Input: part model. Units: mm. Frame: model coordinates. Face numbers are marked on the shaded views. A direction names the side the tool comes from. Round coordinates to 2 decimals unless told otherwise and drop trailing zeros. Loops run counter-clockwise (first coordinate to the right, second up) from the corner with the lowest first, then second, coordinate; pieces in that order, holes last. Notation, with made-up numbers: (82, -31) - (99, -31) arc R33 ccw to (99, 7) - close; hole circle Ø9 at (18.25, -15). An arc over 180 degrees is marked (long way). One line per question, with ' | ' between items. Start each with the question number.
Item 1: Draft query along X for the marked faces 1, 2 and 3. Return one class per face: pulls with the +X half, pulls with the -X half, needs draft (parallel to the pull), parting line crosses it, or undercut.
Item 2: Set-up query: the marked faces 4, 5 and 6. Return all of +Z, -Z, +X, -X, +Y, -Y with unobstructed straight access to the full face (end or side cutting, diameter ignored); none if empty.
Item 3: Material intervals for line 1 along Z through (x, y) = (18.47, -7.75); line 2 along Z through (x, y) = (-38.8, -3.5); line 3 along Z through (x, y) = (28, -3.25), sorted ascending.
Item 4: Section B-B, the plane z = -16.5. Return loops of the section in (x, y).
Item 5: Section C-C, the plane y = -15.5. Return loops of the section in (x, z), plus the area to 3 significant figures.
Item 6: First-contact query: pin 1 (3 mm diameter, centred on x = 36, z = 1, fed in from -Y); pin 2 (1.8 mm diameter, centred on x = -10.5, z = 26.5, fed in from -Y). Flat tips, straight axial feed; report the tip coordinate or a pass-through.
Item 7: Section D-D, the plane y = -5.75. Give the number of separate pieces and of enclosed holes in the cut face, plus the area to 3 significant figures.
Item 8: Section A-A, the plane x = -16. Return loops of the section in (y, z).
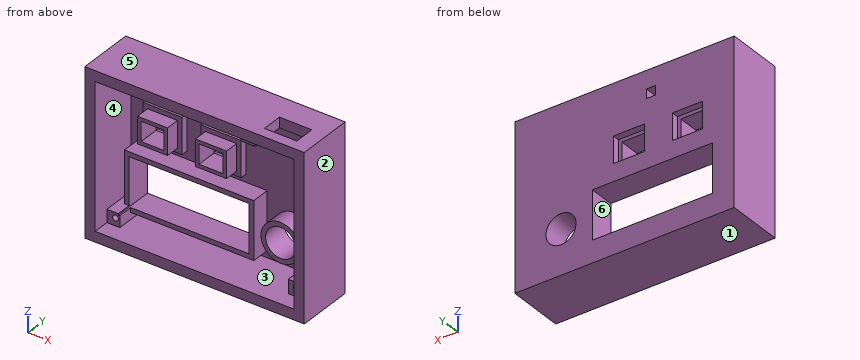
```python
from build123d import *

# Parameters (mm, degrees)
SKETCH1_W             = 13
SKETCH1_H             = 11.5
SKETCH1_W_2           = 13.406613497
SKETCH1_W_3           = 52
SKETCH1_H_2           = 21
SKETCH1_R             = 6.5
BOSS_EXTRUDE1_DEPTH   = 3
SKETCH2_W             = 95
SKETCH2_H             = 71.500049505
BOSS_EXTRUDE2_DEPTH   = 21.5
SKETCH3_R             = 1.25
SKETCH3_W             = 7.478374846
SKETCH3_H             = 5.979454016
SKETCH3_W_2           = 5.973627986
SKETCH3_H_2           = 6.528755861
BOSS_EXTRUDE3_DEPTH   = 14.5
CUT_EXTRUDE1_REACH    = 73.5
SKETCH4_W             = 14
SKETCH4_H             = 9
SKETCH5_R             = 8.5
SKETCH5_R_2           = 6.5
SKETCH5_W             = 56
SKETCH5_H             = 25
SKETCH5_W_2           = 52
SKETCH5_H_2           = 21
BOSS_EXTRUDE4_DEPTH   = 8
SKETCH7_W             = 6
SKETCH7_H             = 6
SKETCH7_W_2           = 4
SKETCH7_H_2           = 4
BOSS_EXTRUDE5_DEPTH   = 13
SKETCH8_W             = 10
SKETCH8_H             = 8.5
BOSS_EXTRUDE6_DEPTH   = 9
SKETCH8_W_2           = 13.406613497
SKETCH8_H_2           = 11.5
SKETCH8_W_3           = 10.406613497
BOSS_EXTRUDE6_2_DEPTH = 9
SKETCH9_W             = 17.406613497
SKETCH9_H             = 15.5
SKETCH9_W_2           = 13.406613497
SKETCH9_H_2           = 11.5
SKETCH9_W_3           = 17
SKETCH9_W_4           = 13
BOSS_EXTRUDE7_DEPTH   = 3
CUT_EXTRUDE2_DEPTH    = 5


with BuildPart() as part:
    # Sketch1 → Boss-Extrude1 (new body)
    with BuildSketch(Plane(origin=(0, 0, 0), x_dir=(1, 0, 0), z_dir=(0, 1, 0))):
        Polygon((48, 35.75), (46, 35.75), (45, 35.75), (-47, 35.75), (-47, 33.75), (-47, -33.75), (-47, -35.750049505), (45, -35.750049505), (46, -35.750049505), (48, -35.750049505), align=None)
        Polygon((-8, -29), (-11, -29), (-14, -29), (-14, -23), (-8, -23), align=None, mode=Mode.SUBTRACT)
        with Locations((-26.716961343, -8)):
            Rectangle(SKETCH1_W, SKETCH1_H, mode=Mode.SUBTRACT)
        with Locations((-1.396693251, -8)):
            Rectangle(SKETCH1_W_2, SKETCH1_H, mode=Mode.SUBTRACT)
        with Locations((-11.6, 15.75)):
            Rectangle(SKETCH1_W_3, SKETCH1_H_2, mode=Mode.SUBTRACT)
        with Locations((28, 16.5)):
            Circle(SKETCH1_R, mode=Mode.SUBTRACT)
    extrude(amount=BOSS_EXTRUDE1_DEPTH)

    # Sketch2 → Boss-Extrude2 (add)
    with BuildSketch(Plane.XZ):
        with Locations((0.5, 2.4752e-05)):
            Rectangle(SKETCH2_W, SKETCH2_H)
        Polygon((41.5, -31.25), (40.5, -31.25), (-42.5, -31.25), (-42.5, 31.25), (40.5, 31.25), (41.5, 31.25), (43.5, 31.25), (43.5, -31.25), align=None, mode=Mode.SUBTRACT)
    extrude(amount=BOSS_EXTRUDE2_DEPTH)

    # Sketch3 → Boss-Extrude3 (add)
    with BuildSketch(Plane.XZ):
        Polygon((-38.8, -25.675777927), (-42.5, -25.675777927), (-42.5, -31.25), (-36.902935229, -31.25), (-36.902935229, -27.93), (-36.902935229, -26.25), (-37.6, -26.25), (-37.6, -25.675777927), align=None)
        with Locations((-38.8, -27.93)):
            Circle(SKETCH3_R, mode=Mode.SUBTRACT)
        with Locations((39.760812577, -28.260272992)):
            Rectangle(SKETCH3_W, SKETCH3_H)
        with Locations((39.43, -27.68)):
            Circle(SKETCH3_R, mode=Mode.SUBTRACT)
        with Locations((18.554223867, 27.98562207)):
            Rectangle(SKETCH3_W_2, SKETCH3_H_2)
        with Locations((18.47, 27.69)):
            Circle(SKETCH3_R, mode=Mode.SUBTRACT)
    extrude(amount=BOSS_EXTRUDE3_DEPTH)

    # Sketch4 → Cut-Extrude1 (cut, up to next)
    with BuildSketch(Plane.XY.offset(35.750049505), mode=Mode.PRIVATE) as cut_extrude1_sk1:
        with Locations((34.5, -12.5)):
            Rectangle(SKETCH4_W, SKETCH4_H)
    cut_extrude1_tool1 = extrude(cut_extrude1_sk1.sketch, amount=-CUT_EXTRUDE1_REACH, mode=Mode.PRIVATE) & part.part
    add(cut_extrude1_tool1.solids().sort_by_distance((34.5, -12.5, 35.75005))[0], mode=Mode.SUBTRACT)

    # Sketch5 → Boss-Extrude4 (add)
    with BuildSketch(Plane.XZ):
        with Locations((28, -16.5)):
            Circle(SKETCH5_R)
        with Locations((28, -16.5)):
            Circle(SKETCH5_R_2, mode=Mode.SUBTRACT)
        with Locations((-11.6, -15.75)):
            Rectangle(SKETCH5_W, SKETCH5_H)
        with Locations((-11.6, -15.75)):
            Rectangle(SKETCH5_W_2, SKETCH5_H_2, mode=Mode.SUBTRACT)
    extrude(amount=BOSS_EXTRUDE4_DEPTH)

    # Sketch7 → Boss-Extrude5 (add)
    with BuildSketch(Plane(origin=(0, 3, 0), x_dir=(1, 0, 0), z_dir=(0, 1, 0))):
        with Locations((-11, -26)):
            Rectangle(SKETCH7_W, SKETCH7_H)
        with Locations((-11, -26)):
            Rectangle(SKETCH7_W_2, SKETCH7_H_2, mode=Mode.SUBTRACT)
    extrude(amount=-BOSS_EXTRUDE5_DEPTH)



with BuildPart() as body_2:
    # Sketch8 → Boss-Extrude6 (new body)
    with BuildSketch(Plane.XZ):
        Polygon((-33.216961343, 12.25), (-33.216961343, 2.25), (-20.216961343, 2.25), (-20.216961343, 12.25), (-20.216961343, 13.75), (-33.216961343, 13.75), align=None)
        with Locations((-26.716961343, 8)):
            Rectangle(SKETCH8_W, SKETCH8_H, mode=Mode.SUBTRACT)
    extrude(amount=BOSS_EXTRUDE6_DEPTH)


with BuildPart() as body_3:
    # Sketch8 → Boss-Extrude6 2 (new body)
    with BuildSketch(Plane.XZ):
        with Locations((-1.396693251, 8)):
            Rectangle(SKETCH8_W_2, SKETCH8_H_2)
        with Locations((-1.396693252, 8)):
            Rectangle(SKETCH8_W_3, SKETCH8_H, mode=Mode.SUBTRACT)
    extrude(amount=BOSS_EXTRUDE6_2_DEPTH)


with BuildPart() as part_1:
    add(part.part)

    add(body_2.part)  # Boss-Extrude7 merges body 2

    add(body_3.part)  # Boss-Extrude7 merges body 3
    # Sketch9 → Boss-Extrude7 (add)
    with BuildSketch(Plane.XZ):
        with Locations((-1.396693252, 8)):
            Rectangle(SKETCH9_W, SKETCH9_H)
        with Locations((-1.396693251, 8)):
            Rectangle(SKETCH9_W_2, SKETCH9_H_2, mode=Mode.SUBTRACT)
        with Locations((-26.716961343, 8)):
            Rectangle(SKETCH9_W_3, SKETCH9_H)
        with Locations((-26.716961343, 8)):
            Rectangle(SKETCH9_W_4, SKETCH9_H_2, mode=Mode.SUBTRACT)
    extrude(amount=BOSS_EXTRUDE7_DEPTH)

    # Sketch10 → Cut-Extrude2 (cut)
    with BuildSketch(Plane.XZ.offset(8)):
        with BuildLine():
            Line((-39.6, -28.25), (-39.6, -26.969531364))
            ThreePointArc((-39.6, -26.969531364), (-38.127998072, -26.876001229), (-37.591654023, -28.25))
            Line((-37.591654023, -28.25), (-39.6, -28.25))
        make_face()
    extrude(amount=-CUT_EXTRUDE2_DEPTH, mode=Mode.SUBTRACT)


solid = part_1.part
```
Return value:
1) face 1: needs draft | face 2: pulls with the +X half | face 3: undercut
2) face 4: -Y | face 5: +Z, +X, -X, +Y, -Y | face 6: +Y, -Y
3) line 1: -35.75 to -31.25, 24.72 to 26.44, 28.94 to 35.75 | line 2: -35.75 to -29.18, -26.68 to -3.25, 31.25 to 35.75 | line 3: -35.75 to -31.25, -25 to -23, -10 to -8, 31.25 to 35.75
4) outline: (-47, -21.5) - (-42.5, -21.5) - (-42.5, 0) - (-39.6, 0) - (-39.6, -8) - (-37.6, -8) - (-37.6, 3) - (-47, 3) - close; (14.4, -8) - (16.4, -8) - (16.4, 0) - (19.5, 0) - (19.5, -8) - (21.5, -8) - (21.5, 3) - (14.4, 3) - close; (34.5, -8) - (36.5, -8) - (36.5, 0) - (43.5, 0) - (43.5, -21.5) - (48, -21.5) - (48, 3) - (34.5, 3) - close
5) outline: (-47, -35.75) - (48, -35.75) - (48, 35.75) - (41.5, 35.75) - (41.5, 31.25) - (43.5, 31.25) - (43.5, -31.25) - (-42.5, -31.25) - (-42.5, 31.25) - (27.5, 31.25) - (27.5, 35.75) - (-47, 35.75) - close | area: 1,350 mm2
6) pin 1: y = 0 | pin 2: through
7) separate pieces: 5 | enclosed holes: 9 | area: 2,060 mm2
8) outline: (-21.5, -35.75) - (3, -35.75) - (3, -26.25) - (-8, -26.25) - (-8, -28.25) - (0, -28.25) - (0, -31.25) - (-21.5, -31.25) - close; (-21.5, 31.25) - (0, 31.25) - (0, -3.25) - (-8, -3.25) - (-8, -5.25) - (3, -5.25) - (3, 35.75) - (-21.5, 35.75) - close
